from build123d import *

# Parameters (mm, degrees)
BOSS_EXTRUDE1_DEPTH      = 50
CUT_EXTRUDE1_DEPTH       = 22
M8_CLEARANCE_HOLE1_D     = 9
M8_CLEARANCE_HOLE1_DEPTH = 30
M8_CLEARANCE_HOLE1_TIP   = 2.703872786
SKETCH6_W                = 21
SKETCH6_H                = 10
BOSS_EXTRUDE2_DEPTH      = 2.5
FILLET1_R                = 1
M5_CLEARANCE_HOLE1_D     = 5.5


with BuildPart() as part:
    # Sketch1 → Boss-Extrude1 (new body)
    with BuildSketch(Plane.XY):
        Polygon((0.253520576, 50), (5.253520576, 50), (5.253520576, 2.5), (16.253520576, 2.5), (16.253520576, 50), (21.253520576, 50), (21.253520576, 0), (0.253520576, 0), align=None)
    extrude(amount=BOSS_EXTRUDE1_DEPTH)

    # Sketch2 → Cut-Extrude1 (cut, through all)
    with BuildSketch(Plane(origin=(21.253520576, 0, 0), x_dir=(0, 0, -1), z_dir=(1, 0, 0))):
        with BuildLine():
            Line((-50, 35), (-50, 50))
            Line((-50, 50), (0, 50))
            Line((0, 50), (0, 35))
            ThreePointArc((0, 35), (-25, 40), (-50, 35))
        make_face()
    extrude(amount=-CUT_EXTRUDE1_DEPTH, mode=Mode.SUBTRACT)

    # M8 Clearance Hole1
    with Locations(Plane(origin=(21.253520576, 0, 0), x_dir=(0, 0, -1), z_dir=(1, 0, 0))):
        with Locations((-25, 30)):
            Hole(M8_CLEARANCE_HOLE1_D / 2, depth=M8_CLEARANCE_HOLE1_DEPTH)
            with Locations((0, 0, -(M8_CLEARANCE_HOLE1_DEPTH + M8_CLEARANCE_HOLE1_TIP / 2))):  # 118° drill point
                Cone(0, M8_CLEARANCE_HOLE1_D / 2, M8_CLEARANCE_HOLE1_TIP, mode=Mode.SUBTRACT)

    # Sketch6 → Boss-Extrude2 (add)
    with BuildSketch(Plane.XZ):
        with Locations((10.753520576, -5)):
            Rectangle(SKETCH6_W, SKETCH6_H)
        with Locations((10.753520576, 55)):
            Rectangle(SKETCH6_W, SKETCH6_H)
    extrude(amount=-BOSS_EXTRUDE2_DEPTH)

    # Fillet1
    fillet1_edges = [part.edges().sort_by_distance(p)[0] for p in [
        (5.253520576, 2.5, 25),
        (16.253520576, 2.5, 25),
        (2.753520576, 2.5, 0),
        (18.753520576, 2.5, 0),
        (18.753520576, 2.5, 50),
        (2.753520576, 2.5, 50),
    ]]
    fillet(fillet1_edges, radius=FILLET1_R)

    # M5 Clearance Hole1 (through all)
    with Locations(Plane(origin=(0, 2.5, 0), x_dir=(1, 0, 0), z_dir=(0, 1, 0))):
        with Locations((5.253520576, -55), (16.253520576, -55), (5.253520576, 5), (16.253520576, 5)):
            Hole(M5_CLEARANCE_HOLE1_D / 2)


solid = part.part
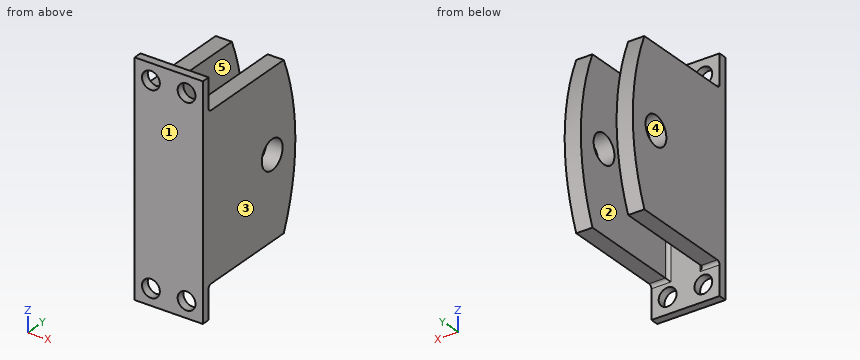
Source: CAD feature listing. Evaluate the final solid. Frame: model axes, mm. Face numbers are marked on the shaded views. A direction names the side the tool comes from. Coordinates: 2 decimals unless noted, no trailing zeros. Loops run counter-clockwise (first coordinate to the right, second up) from the corner with the lowest first, then second, coordinate; pieces in that order, holes last. Notation, with made-up numbers: (39.25, 33) - (63.25, 33) arc R25 cw to (63.25, 62) - close; hole circle Ø11 at (34.25, -25.5). An arc over 180 degrees is marked (long way). One line per question, with ' | ' between items.
1) Line query: line 1 along X through (y, z) = (17, 2); line 2 along X through (y, z) = (1.95, 55); line 3 along Z through (x, y) = (3.5, 16.5). Output: solid intervals per line, ascending.
Report:
line 1: x = 0.25 to 5.25, 16.25 to 21.25 | line 2: x = 0.25 to 2.5, 8 to 13.5, 19 to 21.25 | line 3: z = 0 to 50
2) Section D-D, the plane z = -5. Return loops of the section in (x, y), then the cut area to 3 significant figures.
Report:
outline: (0.25, 0) - (2.5, 0) - (2.5, 2.5) - (0.25, 2.5) - close; (8, 0) - (13.5, 0) - (13.5, 2.5) - (8, 2.5) - close; (19, 0) - (21.25, 0) - (21.25, 2.5) - (19, 2.5) - close | area: 25.0 mm²
3) First-contact query: P1, Ø4, axis at x = 4, y = 14, coming from the -Z side; P2, Ø7, axis at x = 5.25, z = -5, coming from the -Y side; P3, Ø6, axis at x = 12, z = 32, coming from the +Y side; P4, Ø2.5, axis at x = 19.5, y = 19.5, coming from the +Z side. Flat tips, straight axial feed; report the tip coordinate or a pass-through.
Report:
P1: stops at z = 0 | P2: stops at y = 0 | P3: stops at y = 2.5 | P4: stops at z = 50
4) Section C-C, the plane y = 30. Return loops of the section in (x, z).
Report:
outline: (0.25, 0) - (5.25, 0) - (5.25, 20.5) - (0.25, 20.5) - close; (0.25, 29.5) - (5.25, 29.5) - (5.25, 50) - (0.25, 50) - close; (16.25, 0) - (21.25, 0) - (21.25, 20.5) - (16.25, 20.5) - close; (16.25, 29.5) - (21.25, 29.5) - (21.25, 50) - (16.25, 50) - close
5) Pull-direction query (X, two-part tool) for the marked faces 1, 2 and 3; classes: released by +X, released by -X, zero draft, split by the parting line, or undercut.
Report:
face 1: zero draft | face 2: undercut | face 3: released by +X
6) Set-up query: the marked faces 4 and 5. Return all of +Z, -Z, +X, -X, +Y, -Y with unobstructed straight access to the full face (end or side cutting, diameter ignored); none if empty.
Report:
face 4: +X, -X | face 5: +Z, -Z, +Y
7) Section B-B, the plane y = 6.5. Return loops of the section in (x, z).
Report:
outline: (0.25, 0) - (5.25, 0) - (5.25, 50) - (0.25, 50) - close; (16.25, 0) - (21.25, 0) - (21.25, 50) - (16.25, 50) - close
8) Section A-A, the plane z = 25. Return loops of the section in (x, y), then the cut area to 3 significant figures.
Report:
outline: (0.25, 0) - (21.25, 0) - (21.25, 25.5) - (16.25, 25.5) - (16.25, 3.5) arc R1 cw to (15.25, 2.5) - (6.25, 2.5) arc R1 cw to (5.25, 3.5) - (5.25, 25.5) - (0.25, 25.5) - close; (0.25, 34.5) - (5.25, 34.5) - (5.25, 40) - (0.25, 40) - close; (16.25, 34.5) - (21.25, 34.5) - (21.25, 40) - (16.25, 40) - close | area: 338 mm²
